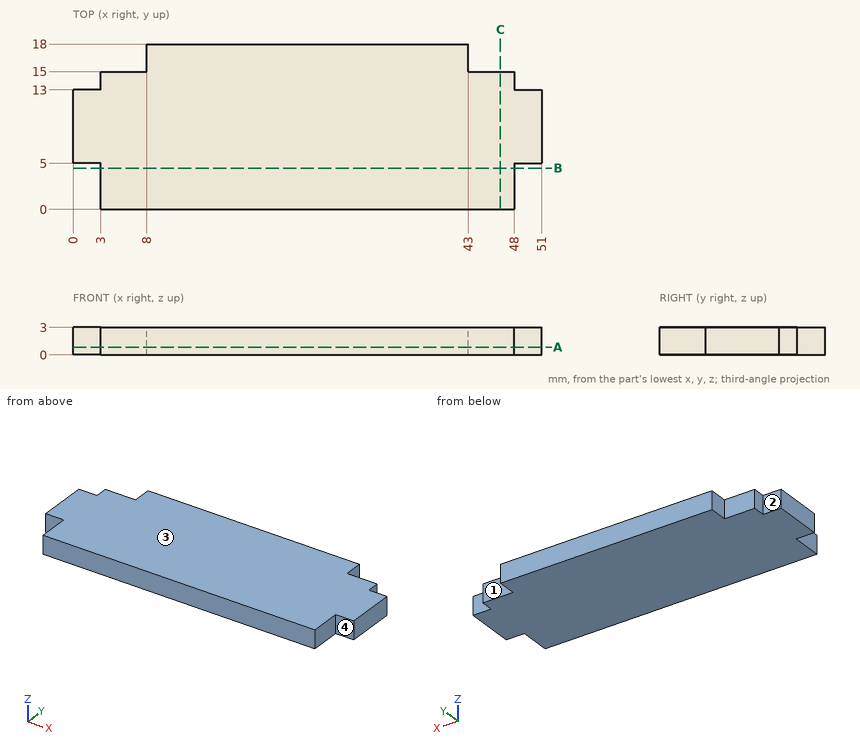
Print and shaded views of the part. All mm, measured from the part's lowest x, y and z. A direction names the side the tool comes from. Round coordinates to 2 decimals unless told otherwise and drop trailing zeros. Write each loop counter-clockwise with the first axis right and the second up, starting at its lowest first coordinate (ties: lowest second). Pieces come first, ordered by that corner, then holes. Notation, with made-up numbers: (35, -28.5) - (80, -28.5) arc R34 ccw to (80, 1.5) - close; hole circle Ø2 at (23, -12.5). An arc over 180 degrees is marked (long way). Write each question's results on one line, items separated by ' | '. Start each with the question number.
Item 1: Drop flat-ended pins along their axis: P1, Ø0.9, axis at y = 3.5, z = 2, coming from the +X side; P2, Ø0.6, axis at y = 14.5, z = 1, coming from the -X side; P3, Ø10, axis at x = 32, y = 11, coming from the -Z side; P4, Ø0.9, axis at x = 46.5, z = 1.5, coming from the +Y side. Give the stop position or say it passes through.
Item 2: Wall check: L1, parallel to X at y = 13.5, z = 1.7; L2, parallel to Y at x = 45.5, z = 0.45; L3, parallel to X at y = 15.5, z = 1.4. Give the ranges that are in metal, low to high. Write a range as [from, to].
Item 3: Saw through at A-A (z = 0.85). Write the cut outline in (x, y).
Item 4: Saw through at C-C (x = 46.5). Write the cut outline in (y, z), and give its area (3 significant figures).
Item 5: Which spindle directions (+Z, -Z, +X, -X, +Y, -Y) get a long thin tool onto all of the face, cutting with end or side? Do the marked faces 1, 2, 3 and 4. Say none if no direction does.
Item 6: Saw through at B-B (y = 4.5). Write the cut outline in (x, z), and give its area (3 significant figures).
Results are:
1) P1: stops at x = 48 | P2: stops at x = 3 | P3: stops at z = 0 | P4: stops at y = 15
2) L1: x = [3, 48] | L2: y = [0, 15] | L3: x = [8, 43]
3) outline: (0, 5) - (3, 5) - (3, 0) - (48, 0) - (48, 5) - (51, 5) - (51, 13) - (48, 13) - (48, 15) - (43, 15) - (43, 18) - (8, 18) - (8, 15) - (3, 15) - (3, 13) - (0, 13) - close
4) outline: (0, 0) - (15, 0) - (15, 3) - (0, 3) - close | area: 45.0 mm²
5) face 1: +Z, -Z, +X, +Y | face 2: +Z, -Z, -X, +Y | face 3: +Z, +X, -X, +Y, -Y | face 4: +Z, -Z, +X, -Y
6) outline: (3, 0) - (48, 0) - (48, 3) - (3, 3) - close | area: 135 mm²
